Here's how the part is built. I have some questions about the finished solid (model axes, mm). Face numbers are marked on the shaded views. Give positions to 0.01 mm unless a question says otherwise; leave off trailing zeros. Order: outer loops, then holes, each group sorted by start corner. A loop starts at its lowest first (then second) coordinate and runs counter-clockwise, first axis right, second up. Notation, with made-up numbers: (75, 59) - (122, 59) arc R13 ccw to (122, 67) - close; hole circle Ø1 at (-40, 71). An arc over 180 degrees is marked (long way). One line per question, with ' | ' between items.
Autodesk Inventor part; units mm, degrees
ref_plane "YZ Plane" through (0, 0, 0) normal (1, 0, 0) x (0, 1, 0)
ref_plane "XZ Plane" through (0, 0, 0) normal (0, 1, 0) x (-1, 0, 0)
ref_plane "XY Plane" through (0, 0, 0) normal (0, 0, 1) x (1, 0, 0)
sketch "Sketch5" plane through (0, 0, 0) normal (0, 1, 0) x (-1, 0, 0)
  line L0 (9.5203, 12.3105) -> (-50.4797, 12.3105)
  line L1 (-50.4797, 12.3105) -> (-50.4797, -27.1895)
  line L2 (-50.4797, -27.1895) -> (9.5203, -27.1895)
  line L3 (9.5203, -27.1895) -> (9.5203, 12.3105)
  line L4 (-33.3579, -22.4395) -> (-31.3579, -22.4395)
  line L5 (-31.3579, -22.4395) -> (-31.3579, 7.5605)
  line L6 (-31.3579, 7.5605) -> (-33.3579, 7.5605)
  line L7 (-33.3579, 7.5605) -> (-33.3579, -22.4395)
  line L8 (8.0203, 7.5605) -> (6.0203, 7.5605)
  line L9 (6.0203, 7.5605) -> (6.0203, -22.3395)
  line L10 (6.0203, -22.3395) -> (8.0203, -22.3395)
  line L11 (8.0203, -22.3395) -> (8.0203, 7.5605)
  circle A0 centre (2.9203, -20.5895) radius 1.5
  circle A1 centre (2.9203, 5.7105) radius 1.5
  circle A2 centre (-34.8579, -24.6895) radius 1.5
  circle A3 centre (-34.8579, 9.8105) radius 1.5
  line L12 (-28.3579, 10.8105) -> (1.6421, 10.8105)
  line L13 (1.6421, 10.8105) -> (1.6421, 8.8105)
  line L14 (1.6421, 8.8105) -> (-28.3579, 8.8105)
  line L15 (-28.3579, 8.8105) -> (-28.3579, 10.8105)
  line L16 (-29.8579, -23.6895) -> (0.1421, -23.6895)
  line L17 (0.1421, -23.6895) -> (0.1421, -25.6895)
  line L18 (0.1421, -25.6895) -> (-29.8579, -25.6895)
  line L19 (-29.8579, -25.6895) -> (-29.8579, -23.6895)
  line L20 (-50.4797, 12.3105) -> (-48.4797, 12.3105)
  line L21 (-48.4797, 12.3105) -> (-48.4797, 10.3105)
  line L22 (-48.4797, 10.3105) -> (-50.4797, 10.3105)
  line L23 (-50.4797, 10.3105) -> (-50.4797, 12.3105)
  point P0 (0, 0)
  point P1 (-29.8579, -24.6895)
  dimension "d9" = 60
  dimension "d10" = 39.5
  dimension "d24" = 2
  dimension "d27" = 4.75
  dimension "d29" = 2
  dimension "d31" = 1.5
  dimension "d32" = 4.75
  dimension "d33" = 4.85
  dimension "d40" = 3
  dimension "d41" = 6.6
  dimension "d42" = 6.6
  dimension "d43" = 3
  dimension "d44" = 6.6
  dimension "d45" = 6.6
  dimension "d46" = 3
  dimension "d47" = 2.5
  dimension "d49" = 3
  dimension "d50" = 2.5
  dimension "d59" = 35
  dimension "d62" = 1.5
  dimension "d66" = 35
  dimension "d73" = 1.5
  dimension "d74" = 30
  dimension "d75" = 5
  dimension "d76" = 2
  dimension "d77" = 5
  dimension "d78" = 1.5
  dimension "d79" = 30
  dimension "d80" = 2
  dimension "d81" = 2
  dimension "d82" = 2
extrude "Extrusion8" add sketch "Sketch5" against normal blind 1.5 contours L3 L2 L1 L22 L21 L0 | L21 L22 L1 L0 | L7 L6 L5 L4 | L11 L10 L9 L8 | A0 | A1 | A2 | A3 | L12 L13 L14 L15 | L16 L17 L18 L19
extrude "Extrusion9" add sketch "Sketch5" along normal blind 3.5 contours L21 L22 L1 L0 | L7 L6 L5 L4 | L11 L10 L9 L8 | L12 L13 L14 L15 | L16 L17 L18 L19
extrude "Extrusion10" add sketch "Sketch5" along normal blind 6 contours A0 | A1 | A2 | A3
properties part number "RFID-RC522 Holder 3.3"
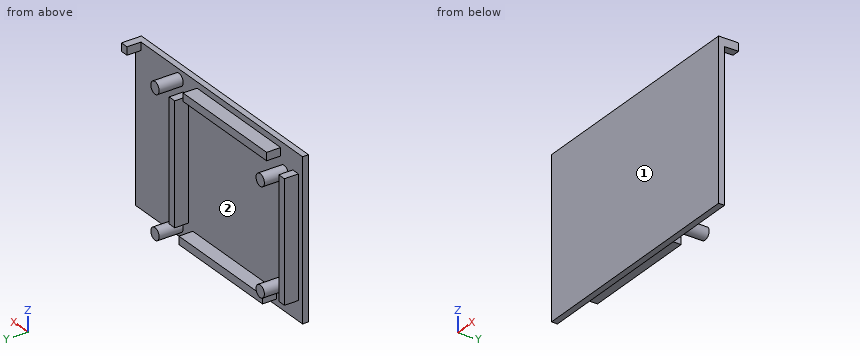
1) I'm going to push flat-ended pins straight in: P1, Ø2, axis at x = -7, y = 2, coming from the -Z side; P2, Ø1, axis at x = 12, y = 2, coming from the +Z side; P3, Ø3, axis at x = 1.5, y = 0.5, coming from the -Z side; P4, Ø1, axis at x = 32.5, y = 2.5, coming from the +Z side. Where does each tip first touch, or does it pass through?
Model answer:
P1: stops at z = -22.34 | P2: stops at z = 10.81 | P3: stops at z = -27.19 | P4: stops at z = 7.56
2) Please list where these lines run through material, in increasing order: L1, parallel to Z at x = 5, y = 2.5; L2, parallel to X at y = 1.75, z = -15; L3, parallel to X at y = 1.5, z = 7.
Model answer:
L1: z = -25.69 to -23.69, 8.81 to 10.81 | L2: x = -8.02 to -6.02, 31.36 to 33.36 | L3: x = -8.02 to -6.02, -3.69 to -2.15, 31.36 to 33.36
3) Thinking about a two-plate mould opening in Z: for the marked faces 1 and 2, which applies, +Z half, -Z half, draft (parallel to the pull), parting line (faces both ways), or undercut?
Model answer:
face 1: draft | face 2: undercut
4) I want a section at B-B (z = -9.5). List the corners of the cut face in (x, y) for me, plus the area to 3 significant figures.
Model answer:
outline: (-9.52, -1.5) - (50.48, -1.5) - (50.48, 0) - (33.36, 0) - (33.36, 3.5) - (31.36, 3.5) - (31.36, 0) - (-6.02, 0) - (-6.02, 3.5) - (-8.02, 3.5) - (-8.02, 0) - (-9.52, 0) - close | area: 104 mm2
5) I want a section at D-D (z = -20). List the corners of the cut face in (x, y) for me, plus the area to 3 significant figures.
Model answer:
outline: (-9.52, -1.5) - (50.48, -1.5) - (50.48, 0) - (33.36, 0) - (33.36, 3.5) - (31.36, 3.5) - (31.36, 0) - (-1.54, 0) - (-1.54, 6) - (-4.3, 6) - (-4.3, 0) - (-6.02, 0) - (-6.02, 3.5) - (-8.02, 3.5) - (-8.02, 0) - (-9.52, 0) - close | area: 121 mm2
6) I want a section at C-C (x = 6). List the corners of the cut face in (y, z) for me, plus the area to 4 significant figures.
Model answer:
outline: (-1.5, -27.19) - (0, -27.19) - (0, -25.69) - (3.5, -25.69) - (3.5, -23.69) - (0, -23.69) - (0, 8.81) - (3.5, 8.81) - (3.5, 10.81) - (0, 10.81) - (0, 12.31) - (-1.5, 12.31) - close | area: 73.25 mm2
7) I want a section at A-A (y = 2). State how many separate pieces and enclosed holes the cut face has, plus the area to 3 significant figures.
Model answer:
separate pieces: 9 | enclosed holes: 0 | area: 272 mm2
